The listing builds one solid part. Answer for the finished solid, in the listing's coordinates (mm). Round coordinates to 2 decimals unless told otherwise and drop trailing zeros. Order: outer loops, then holes, each group sorted by start corner. A loop starts at its lowest first (then second) coordinate and runs counter-clockwise, first axis right, second up. Notation, with made-up numbers: (-4, -28) - (45, -28) arc R26 cw to (45, -11) - close; hole circle Ø7 at (32.25, -2). An arc over 180 degrees is marked (long way). One line per item, written item: value. Start each with the question number.
1. Section C-C, the plane y = -4 is taken. Give the vertices of the cut face in (x, z), then the cut area to 3 significant figures.
2. Section B-B, the plane x = -25.4 is taken. Give the vertices of the cut face in (y, z), then the cut area to 3 significant figures.
3. Section A-A, the plane x = 0 is taken. Give the vertices of the cut face in (y, z), then the cut area to 3 significant figures.
4. For a pull along X with two mould halves and no side action, classify faces 1 (the flat face through (31.75, 0, 3)), 2 (the flat face through (-31.75, 0, 3)), 3 (the cylindrical face through (16.7, -1, 3.1)) as released by +X, released by -X, zero draft, split by the parting line, or undercut.
5. Straight lines are drawn through the part: line 1 (Y direction, x = -25.4, z = 3.25); line 2 (Y direction, x = 19.05, z = 2.25); line 3 (X direction, y = 27.5, z = 1). For each, find the intervals that lie inside material, in ascending order.
from build123d import *

# Parameters (mm, degrees)
SKETCH1_W              = 63.5
SKETCH1_H              = 63.5
BOSS_EXTRUDE1_DEPTH    = 6.35
F_10_CLEARANCE_HOLE3_D = 5.1054
F_10_CLEARANCE_HOLE2_D = 5.1054
HOLE1_D                = 12.7


with BuildPart() as part:
    # Sketch1 → Boss-Extrude1 (new body)
    with BuildSketch(Plane.XY):
        Rectangle(SKETCH1_W, SKETCH1_H)
    extrude(amount=BOSS_EXTRUDE1_DEPTH)

    # #10 Clearance Hole3 (through all)
    with Locations(Plane.XY.offset(6.35)):
        with Locations((-25.4, 25.4), (25.4, -25.4), (-25.4, -25.4), (25.4, 25.4)):
            Hole(F_10_CLEARANCE_HOLE3_D / 2)

    # #10 Clearance Hole2 (through all)
    with Locations(Plane.XY.offset(6.35)):
        with Locations((-19.05, 0), (19.05, 0)):
            Hole(F_10_CLEARANCE_HOLE2_D / 2)

    # Hole1 (through all)
    with Locations(Plane.XY.offset(6.35)):
        with Locations((0, -8.3566)):
            Hole(HOLE1_D / 2)


solid = part.part
Answer list:
1. outline: (-31.75, 0) - (-4.62, 0) - (-4.62, 6.35) - (-31.75, 6.35) - close; (4.62, 0) - (31.75, 0) - (31.75, 6.35) - (4.62, 6.35) - close
1. area: 345 mm²
2. outline: (-31.75, 0) - (-27.95, 0) - (-27.95, 6.35) - (-31.75, 6.35) - close; (-22.85, 0) - (22.85, 0) - (22.85, 6.35) - (-22.85, 6.35) - close; (27.95, 0) - (31.75, 0) - (31.75, 6.35) - (27.95, 6.35) - close
2. area: 338 mm²
3. outline: (-31.75, 0) - (-14.71, 0) - (-14.71, 6.35) - (-31.75, 6.35) - close; (-2.01, 0) - (31.75, 0) - (31.75, 6.35) - (-2.01, 6.35) - close
3. area: 323 mm²
4. face 1: released by +X
4. face 2: released by -X
4. face 3: undercut
5. line 1: y = -31.75 to -27.95, -22.85 to 22.85, 27.95 to 31.75
5. line 2: y = -31.75 to -2.55, 2.55 to 31.75
5. line 3: x = -31.75 to -26.85, -23.95 to 23.95, 26.85 to 31.75
